```python
from build123d import *

# Parameters (mm, degrees)
BOSS_EXTRUDE1_DEPTH        = 6.35
F_9_0_196_DIAMETER_HOLE1_D = 4.9784
FILLET1_R                  = 6.35


with BuildPart() as part:
    # Sketch1 → Boss-Extrude1 (new body)
    with BuildSketch(Plane.YZ):
        with BuildLine():
            Line((-13.06131899, 62.142191354), (-120.903176517, 112.429675389))
            ThreePointArc((-120.903176517, 112.429675389), (-161.186470776, 35.734180261), (-157.090324336, -50.8))
            Line((-157.090324336, -50.8), (-38.1, -50.8))
            ThreePointArc((-38.1, -50.8), (-61.994796452, 13.743915485), (-13.06131899, 62.142191354))
        make_face()
    extrude(amount=BOSS_EXTRUDE1_DEPTH)

    # #9 (0.196) Diameter Hole1 (through all)
    with Locations(Plane.YZ.offset(6.35)):
        with Locations((-116.264496524, 96.253723813), (-47.203843152, 64.050212269)):
            Hole(F_9_0_196_DIAMETER_HOLE1_D / 2)

    # Fillet1
    fillet1_edges = [part.edges().sort_by_distance(p)[0] for p in [
        (3.175, -120.903176517, 112.429675389),
        (3.175, -13.06131899, 62.142191354),
        (3.175, -38.1, -50.8),
        (3.175, -157.090324336, -50.8),
    ]]
    fillet(fillet1_edges, radius=FILLET1_R)


solid = part.part
```
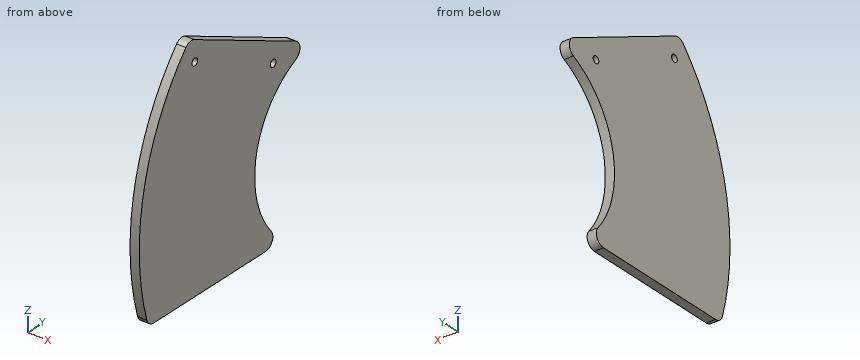
Geometry check sheet. Reference: the model listing, model coordinates, mm. Round coordinates to 2 decimals unless told otherwise and drop trailing zeros. Order: outer loops, then holes, each group sorted by start corner. A loop starts at its lowest first (then second) coordinate and runs counter-clockwise, first axis right, second up. Notation, with made-up numbers: M 86.25,26 L 103.25,26 A23 ccw 103.25,44 Z; hole C 48,74 d8. An arc over 180 degrees is marked long. Answer as CSV lines item,"result".
1) Sectioned sample at A-A on x = 3.5. Record the cut outline in (y, z), and give its area (3 significant figures).
Entries:
outline,"M -158.5,-46.23 A6.35 ccw -152.4,-50.8 L -53.88,-50.8 A6.35 ccw -48.98,-40.41 A63.5 cw -27.32,57.32 A6.35 ccw -27.36,68.81 L -116.65,110.45 A6.35 ccw -124.11,108.88 A165.1 ccw Z; hole C -116.26,96.25 d4.98; hole C -47.2,64.05 d4.98"
area,"15,800 mm2"
2) Gauge pin test, flat ends, axial feed: pin 1 Ø4 at (y, z) = (-116.26, 96.25) entering from -X; pin 2 Ø3 at (x, y) = (4.5, -61.5) entering from +Z. Record the tip position at first contact, or that the pin passes through.
Entries:
pin 1,"through"
pin 2,"z = 85.43"
3) Sectioned sample at B-B on y = -101. Record the cut outline in (x, z), and give its area (3 significant figures).
Entries:
outline,"M 0,-50.8 L 6.35,-50.8 L 6.35,103.15 L 0,103.15 Z"
area,"978 mm2"
4) Thickness scan on probe 1 along Y at (x, z) = (5.75, -2); probe 2 along Z at (x, y) = (5, -90.5); probe 3 along Z at (x, y) = (3.5, -70). Record the ranges inside material, lowest first. Write a range as [from, to].
Entries:
probe 1,"[-165.09, -63.47]"
probe 2,"[-50.8, 98.25]"
probe 3,"[-50.8, 88.69]"
5) Sectioned sample at C-C on z = 73.5. Record the cut outline in (x, y), and give its area (3 significant figures).
Entries:
outline,"M 0,-147.84 L 6.35,-147.84 L 6.35,-37.42 L 0,-37.42 Z"
area,"701 mm2"
